Check sheet for the modelled part. Datum: model origin and axes. Units: mm. Round coordinates to 2 decimals unless told otherwise and drop trailing zeros. Write each loop counter-clockwise with the first axis right and the second up, starting at its lowest first coordinate (ties: lowest second). Pieces come first, ordered by that corner, then holes. Notation, with made-up numbers: (-23.5, 64.25) -> (0.5, 64.25) arc R28 cw to (0.5, 102.25) -> close; hole circle Ø10 at (4.25, 27.25). An arc over 180 degrees is marked (long way). Answer as a JSON object with one key per item and string values. Group by question number.
```python
from build123d import *

# Parameters (mm, degrees)
SKETCH4_R           = 2.5
BOSS_EXTRUDE2_DEPTH = 6
SKETCH5_R           = 2.5
CUT_EXTRUDE1_DEPTH  = 27.511142593


with BuildPart() as part:
    # Sketch4 → Boss-Extrude2 (new body)
    with BuildSketch(Plane.XY):
        with BuildLine():
            Line((-9.5, 6.468437336), (12.5, 6.468437336))
            Line((12.5, 6.468437336), (12.5, -6.468437336))
            Line((12.5, -6.468437336), (-9.5, -6.468437336))
            ThreePointArc((-9.5, -6.468437336), (-11.621320344, -5.58975768), (-12.5, -3.468437336))
            Line((-12.5, -3.468437336), (-12.5, 3.468437336))
            ThreePointArc((-12.5, 3.468437336), (-11.621320344, 5.58975768), (-9.5, 6.468437336))
        make_face()
        with Locations(Location((9.5, 0, 0), (0, 0, 180))):
            Circle(SKETCH4_R, mode=Mode.SUBTRACT)
    extrude(amount=BOSS_EXTRUDE2_DEPTH)

    # Sketch5 → Cut-Extrude1 (cut, through all)
    with BuildSketch(Plane.ZY.offset(12.5)):
        with Locations((3.019651732, 0)):
            Circle(SKETCH5_R)
    extrude(amount=-CUT_EXTRUDE1_DEPTH, mode=Mode.SUBTRACT)


solid = part.part
```
(1) Section check A-A on y = 0. Record the cut outline in (x, z).
(2) Scan lines: line 1 along Y through (x, z) = (9.5, 1.05); line 2 along Y through (x, z) = (0, 2.2); line 3 along X through (y, z) = (1.25, 0.8). Record each from-to range of solid material in increasing order.
(3) Section check C-C on x = 0. Record the cut outline in (y, z).
(4) Go/stop test with a flat-tipped pin: pin 1 Ø3 at (x, y) = (9.5, 0) entering from -Z. Record where the tip stops, or that it passes through.
(5) Section check D-D on y = -2.25. Record the cut outline in (x, z), then the cut area to 3 significant figures.
(6) Release check for a two-part mould opening along Y. For faces 1 (the flat face through (2, -6.468, 3)), 2 (the flat face through (0, 0, 6)), 3 (the cylindrical face through (11.65, 2.11, 4.36)), 4 (the cylindrical face through (8, -2, 5)) record: pulls with the +Y half, pulls with the -Y half, needs draft (parallel to the pull), parting line crosses it, or undercut.
(7) Section check B-B on z = 4. Record the cut outline in (x, y), then the cut area to 3 significant figures.
Data:
{
 "1": {"outline": "(-12.5, 0) -> (7, 0) -> (7, 0.52) -> (-12.5, 0.52) -> close; (-12.5, 5.52) -> (7, 5.52) -> (7, 6) -> (-12.5, 6) -> close; (12, 0) -> (12.5, 0) -> (12.5, 0.52) -> (12, 0.52) -> close; (12, 5.52) -> (12.5, 5.52) -> (12.5, 6) -> (12, 6) -> close"},
 "2": {"line 1": "y = -6.47 to -2.5, 2.5 to 6.47", "line 2": "y = -6.47 to -2.36, 2.36 to 6.47", "line 3": "x = -12.5 to 7.33, 11.67 to 12.5"},
 "3": {"outline": "(-6.47, 0) -> (6.47, 0) -> (6.47, 6) -> (-6.47, 6) -> close; hole circle Ø5 at (0, 3.02)"},
 "4": {"pin 1": "passes through"},
 "5": {"outline": "(-12.5, 0) -> (8.41, 0) -> (8.41, 1.93) -> (-12.5, 1.93) -> close; (-12.5, 4.11) -> (8.41, 4.11) -> (8.41, 6) -> (-12.5, 6) -> close; (10.59, 0) -> (12.5, 0) -> (12.5, 1.93) -> (10.59, 1.93) -> close; (10.59, 4.11) -> (12.5, 4.11) -> (12.5, 6) -> (10.59, 6) -> close", "area": "87.2 mm²"},
 "6": {"face 1": "pulls with the -Y half", "face 2": "needs draft", "face 3": "undercut", "face 4": "undercut"},
 "7": {"outline": "(-12.5, -3.47) arc R3 ccw to (-9.5, -6.47) -> (12.5, -6.47) -> (12.5, -2.3) -> (10.48, -2.3) arc R2.5 cw to (8.52, -2.3) -> (-12.5, -2.3) -> close; (-12.5, 2.3) -> (8.52, 2.3) arc R2.5 cw to (10.48, 2.3) -> (12.5, 2.3) -> (12.5, 6.47) -> (-9.5, 6.47) arc R3 ccw to (-12.5, 3.47) -> close", "area": "204 mm²"}
}
